Autodesk Fusion 360 part; units mm, degrees
sketch "Skizze1" plane through (0, 0, 0) normal (0, 1, 0) x (1, 0, 0)
  line L0 (0, 0) -> (12, 0)
  line L1 (12, 0) -> (9.1788, 16)
  line L2 (9.1788, 16) -> (4, 16)
  line L3 (4, 16) -> (4, 10)
  line L4 (4, 10) -> (0, 10)
  line L5 (0, 10) -> (0, 0)
  dimension "d1" = 12
  dimension "d2" = 80
  dimension "d3" = 16
  dimension "d4" = 4
  dimension "d5" = 6
revolve "Drehen1" add sketch "Skizze1" angle 360 about axis through (0, 0, 1.75) along (0, 0, 1)
fillet "Abrundung1" radius 0.4 1 edges at (-11.1879, -4.3394, 0)
fillet "Abrundung2" radius 1 2 edges at (-3.7293, -1.4465, -16) (-8.5576, -3.3192, -16)
Geometry: final body of the model. Coordinates: model frame, mm. A direction names the side the tool comes from. Give positions to 0.01 mm unless a question says otherwise; leave off trailing zeros. Order: outer loops, then holes, each group sorted by start corner. A loop starts at its lowest first (then second) coordinate and runs counter-clockwise, first axis right, second up. Notation, with made-up numbers: (55.25, 88.5) -> (75.25, 88.5) arc R9 ccw to (75.25, 92.5) -> close; hole circle Ø5 at (-4, -19). An arc over 180 degrees is marked (long way). Write each question's results on one line, items separated by ' | '. Start each with the question number.
1) Set-up query: faces 4 (the flat face through (0, 0, 0)), 5 (the flat face through (0, 0, -10)). Return all of +Z, -Z, +X, -X, +Y, -Y with unobstructed straight access to the full face (end or side cutting, diameter ignored); none if empty.
2) Section C-C (z = -4). Return loops of the section in (x, y), then the cut area to 3 significant figures.
3) Section A-A (y = 0). Return loops of the section in (x, z).
4) Draft query along Y for faces 1 (the flat face through (4, -4, -16)), 2 (the conical face through (-8.2, -6.3, -9.4)), 3 (the cylindrical face through (-0.867, -3.905, -12.465)). Return one class per face: pulls with the +Y half, pulls with the -Y half, needs draft (parallel to the pull), parting line crosses it, or undercut.
5) First-contact query: pin 1 (10.5 mm diameter, centred on x = 0, y = 0, fed in from -Z); pin 2 (2.5 mm diameter, centred on x = 1.5, y = -1.5, fed in from -Z); pin 3 (1.5 mm diameter, centred on y = -2.5, z = -7.5, fed in from +X); pin 4 (5 mm diameter, centred on y = -1.5, z = -13.5, fed in from +X). Flat tips, straight axial feed; report the tip coordinate or a pass-through.
6) Line query: line 1 (Y direction, x = 0, z = -13); line 2 (X direction, y = 1, z = -13); line 3 (Z direction, x = -7, y = -4.75). Output: solid intervals per line, ascending. Write a range as from..to.
Calculated:
1) face 4: +Z, +X, -X, +Y, -Y | face 5: -Z
2) outline: circle Ø22.59 at (0, 0) | area: 401 mm2
3) outline: (-11.92, -0.47) -> (-9.32, -15.17) arc R1 ccw to (-8.34, -16) -> (-5, -16) arc R1 ccw to (-4, -15) -> (-4, -10) -> (4, -10) -> (4, -15) arc R1 ccw to (5, -16) -> (8.34, -16) arc R1 ccw to (9.32, -15.17) -> (11.92, -0.47) arc R0.4 ccw to (11.52, 0) -> (-11.52, 0) arc R0.4 ccw to start
4) face 1: needs draft | face 2: parting line crosses it | face 3: undercut
5) pin 1: z = -16 | pin 2: z = -10 | pin 3: x = 10.59 | pin 4: x = 10.01
6) line 1: -9.71..-4, 4..9.71 | line 2: -9.66..-3.87, 3.87..9.66 | line 3: -15.99..0
